from build123d import *


with BuildPart() as part:
    # Szkic1 → Obrót1 (revolve)
    with BuildSketch(Plane.XY, mode=Mode.PRIVATE) as obr_t1_sk:
        Polygon((-2.324733291, 2.132645156), (-2.639292136, 3), (-13.441762305, 3), (-13.907929964, 2.132645156), (-14.17640763, 2.132645156), (-14.589993676, 3), (-14.883717364, 3), (-15.363713775, 2.132645156), (-15.586413954, 2.132645156), (-16, 3), (-17, 3), (-17, 0), (0, 0), (0.327556569, 0), (0.327556569, 3), (0.104856391, 3), (-0.375140021, 2.132645156), (-0.901728995, 2.132645156), (-1.321140788, 3), (-1.695615602, 3), (-2.008291441, 2.132645156), align=None)
    revolve(obr_t1_sk.sketch.rotate(Axis((0.327556569, -3, 0), (-1, 0, 0)), 90), axis=Axis((0.327556569, -3, 0), (-1, 0, 0)))


solid = part.part
Geometry: final body of the model. Coordinates: model frame, mm. A direction names the side the tool comes from. Give positions to 0.01 mm unless a question says otherwise; leave off trailing zeros. Order: outer loops, then holes, each group sorted by start corner. A loop starts at its lowest first (then second) coordinate and runs counter-clockwise, first axis right, second up. Notation, with made-up numbers: (84, 74) -> (135, 74) arc R14 cw to (135, 87) -> close; hole circle Ø2 at (-38, 36.25). An arc over 180 degrees is marked (long way). Answer as a JSON object with one key per item and string values.
Q1. Material intervals for probe 1 along X at (y, z) = (0.75, -4.5); probe 2 along Y at (x, z) = (-6.5, 0); probe 3 along X at (y, z) = (-7.25, 3.5), sorted ascending.
Entries:
{"probe 1": "x = -17 to -15.93, -14.96 to -14.52, -13.52 to -2.59, -1.75 to -1.25, 0.03 to 0.33", "probe 2": "y = -9 to -6, 0 to 3", "probe 3": "x = -17 to -15.76, -15.16 to -14.35, -13.71 to -2.46, -1.87 to -1.08, -0.17 to 0.33"}
Q2. Section A-A (x = -8). Output: boundary loops of the cut face in (y, z), plus the area to 3 significant figures.
Entries:
{"outline": "circle Ø12 at (-3, 0); hole circle Ø6 at (-3, 0)", "area": "84.8 mm^2"}
Q3. First-contact query: pin 1 (2 mm diameter, centred on x = -6.5, z = 3, fed in from +Y); pin 2 (3 mm diameter, centred on x = -12, z = -3, fed in from +Y); pin 3 (1.5 mm diameter, centred on x = -8.5, y = -5.5, fed in from -Z). Flat tips, straight axial feed; report the tip coordinate or a pass-through.
Entries:
{"pin 1": "stops at y = 2.66", "pin 2": "stops at y = 2.81", "pin 3": "stops at z = -5.74"}
Q4. Access query for faces 4 (the flat face through (-17, -2, 3)), 5 (the cylindrical face through (-2.169, 1.554, -2.368)). Directions: +Z, -Z, +X, -X, +Y, -Y. A direction counts if a zero-diameter tool reaches every point of the face in a straight line with its end or side. Return the directions, or none.
Entries:
{"face 4": "+Z, -Z, -X, +Y, -Y", "face 5": "none"}
Q5. Draft query along X for faces 1 (the flat face through (0.328, -6, 1)), 2 (the cylindrical face through (-0.642, 1.554, -2.368)), 3 (the cylindrical face through (-8.21, -3.9, -2.86)). Return one class per face: released by +X, released by -X, zero draft, split by the parting line, or undercut.
Entries:
{"face 1": "released by +X", "face 2": "undercut", "face 3": "zero draft"}
